Geometry check sheet. Reference: the model listing, model coordinates, mm. Face numbers are marked on the shaded views. A direction names the side the tool comes from. Give positions to 0.01 mm unless a question says otherwise; leave off trailing zeros. Loops run counter-clockwise (first coordinate to the right, second up) from the corner with the lowest first, then second, coordinate; pieces in that order, holes last. Notation, with made-up numbers: (-7, 33) -> (15, 33) arc R31 cw to (15, 61) -> close; hole circle Ø7 at (24.25, 66). An arc over 180 degrees is marked (long way). One line per item, written item: value. Start each with the question number.
(1) Scan lines: line 1 along X through (y, z) = (36.5, 28); line 2 along Y through (x, z) = (-22.5, 28); line 3 along Y through (x, z) = (21, 1.5). Record each from-to range of solid material in increasing order. Write a range as from..to.
(2) Tool access check on the marked faces 1, 2 and 3. Record the directions out of +Z, -Z, +X, -X, +Y, -Y that give a thin tool (end or side, any length) a straight path to the whole face; none if there is none.
(3) Draft check along Y on the marked faces 4, 5 and 6. Enter one of: pulls with the +Y half, pulls with the -Y half, needs draft (parallel to the pull), parting line crosses it, or undercut.
(4) Sectioned sample at B-B, the plane y = -69. Record the cut outline in (x, z).
(5) Gauge pin test, flat ends, axial feed: pin 1 Ø4 at (y, z) = (45, 14) entering from +X; pin 2 Ø4 at (x, y) = (-29, 64) entering from +Z; pin 3 Ø12 at (x, y) = (24.5, 66) entering from -Z; pin 4 Ø3 at (x, y) = (-10, 18.5) entering from -Z. Record the tip position at first contact, or that the pin passes through.
(6) Sectioned sample at C-C, the plane y = 1. Record the cut outline in (x, z), then the cut area to 3 significant figures.
(7) Sectioned sample at A-A, the plane x = 109. Record the cut outline in (y, z), then the cut area to 3 significant figures.
from build123d import *

# Parameters (mm, degrees)
F0_W      = 252.4125
F0_H      = 252.4125
F0_W_2    = 100.80625
F0_H_2    = 100.80625
F1_DEPTH  = 25.4
F2_W      = 100.80625
F2_H      = 100.80625
F3_DEPTH  = 6.35
F4_R      = 4
F4_R_2    = 1.7272
F5_DEPTH  = 6.35
F6_W      = 14.3500094
F6_H      = 31.75
F7_DEPTH  = 1.5875
F8_R      = 4
F9_DEPTH  = 6.35
F10_W     = 252.4125
F10_H     = 252.4125
F10_W_2   = 100.80625
F10_H_2   = 100.80625
F10_W_3   = 1.5875
F10_H_3   = 14.3500094
F11_DEPTH = 6.35


with BuildPart() as f1:
    # F0 (on Top) → F1 (new body)
    with BuildSketch(Plane.XY):
        Rectangle(F0_W, F0_H)
        Polygon((12.7, -12.7), (12.7, -119.85625), (-119.85625, -119.85625), (-119.85625, 12.7), (-12.7, 12.7), (-12.7, 119.85625), (119.85625, 119.85625), (119.85625, -12.7), align=None, mode=Mode.SUBTRACT)
        with Locations((69.453125, -69.453125)):
            Rectangle(F0_W_2, F0_H_2, mode=Mode.SUBTRACT)
        with Locations((-69.453125, 69.453125)):
            Rectangle(F0_W_2, F0_H_2, mode=Mode.SUBTRACT)
    extrude(amount=F1_DEPTH)

    # F2 (on face) → F3 (join)
    with BuildSketch(Plane.XY.offset(25.4)):
        Polygon((126.20625, -126.20625), (126.20625, 12.7), (119.85625, 12.7), (119.85625, -12.7), (12.7, -12.7), (12.7, -119.85625), (-12.7, -119.85625), (-12.7, -126.20625), align=None)
        with Locations((69.453125, -69.453125)):
            Rectangle(F2_W, F2_H, mode=Mode.SUBTRACT)
        Polygon((12.7, 126.20625), (-126.20625, 126.20625), (-126.20625, -12.7), (-119.85625, -12.7), (-119.85625, 12.7), (-12.7, 12.7), (-12.7, 119.85625), (12.7, 119.85625), align=None)
        with Locations((-69.453125, 69.453125)):
            Rectangle(F2_W, F2_H, mode=Mode.SUBTRACT)
        Polygon((12.7, 12.7), (12.7, 119.85625), (-12.7, 119.85625), (-12.7, 12.7), (-119.85625, 12.7), (-119.85625, -12.7), (-12.7, -12.7), (-12.7, -119.85625), (12.7, -119.85625), (12.7, -12.7), (119.85625, -12.7), (119.85625, 12.7), align=None)
        Polygon((-119.85625, -12.7), (-126.20625, -12.7), (-126.20625, -126.20625), (-12.7, -126.20625), (-12.7, -119.85625), (-119.85625, -119.85625), align=None)
        Polygon((126.20625, 126.20625), (12.7, 126.20625), (12.7, 119.85625), (119.85625, 119.85625), (119.85625, 12.7), (126.20625, 12.7), align=None)
    extrude(amount=F3_DEPTH)

    # F4 (on face) → F5 (cut, through all)
    with BuildSketch(Plane.YZ.offset(126.20625)):
        with Locations((107.91875, 12.7)):
            Circle(F4_R)
        with Locations((115.8875, 12.7)):
            Circle(F4_R_2)
        with Locations((99.95, 12.7)):
            Circle(F4_R_2)
        with Locations((44.41875, 12.7)):
            Circle(F4_R)
        with Locations((52.3875, 12.7)):
            Circle(F4_R_2)
        with Locations((36.45, 12.7)):
            Circle(F4_R_2)
    extrude(amount=-F5_DEPTH, mode=Mode.SUBTRACT)

    # F6 (on face) → F7 (join)
    with BuildSketch(Plane(origin=(-19.05, 0, 0), x_dir=(0, -1, 0), z_dir=(-1, 0, 0))):
        with Locations((-44.41875, 15.875)):
            Rectangle(F6_W, F6_H)
        with Locations((-107.91875, 15.875)):
            Rectangle(F6_W, F6_H)
    extrude(amount=F7_DEPTH)

    # F8 (on face) → F9 (cut, through all)
    with BuildSketch(Plane.YZ.offset(-12.7)):
        with Locations((44.41875, 12.7)):
            Circle(F8_R)
        with Locations((107.91875, 12.7)):
            Circle(F8_R)
    extrude(amount=-F9_DEPTH, mode=Mode.SUBTRACT)

    # F10 (on face) → F11 (join)
    with BuildSketch(Plane(origin=(0, 0, 0), x_dir=(1, 0, 0), z_dir=(0, 0, -1))):
        Rectangle(F10_W, F10_H)
        Polygon((-119.85625, -19.05), (-19.05, -19.05), (-19.05, -37.2437453), (-19.05, -51.5937547), (-19.05, -100.7437453), (-19.05, -115.0937547), (-19.05, -119.85625), (-119.85625, -119.85625), align=None, mode=Mode.SUBTRACT)
        Polygon((-119.85625, 119.85625), (12.7, 119.85625), (12.7, 12.7), (119.85625, 12.7), (119.85625, -119.85625), (-12.7, -119.85625), (-12.7, -12.7), (-119.85625, -12.7), align=None, mode=Mode.SUBTRACT)
        with Locations((69.453125, 69.453125)):
            Rectangle(F10_W_2, F10_H_2, mode=Mode.SUBTRACT)
        with Locations((69.453125, 69.453125)):
            Rectangle(F10_W_2, F10_H_2)
        Polygon((-19.05, -37.2437453), (-19.05, -19.05), (-119.85625, -19.05), (-119.85625, -119.85625), (-19.05, -119.85625), (-19.05, -115.0937547), (-20.6375, -115.0937547), (-20.6375, -100.7437453), (-19.05, -100.7437453), (-19.05, -51.5937547), (-20.6375, -51.5937547), (-20.6375, -37.2437453), align=None)
        with Locations((-19.84375, -44.41875)):
            Rectangle(F10_W_3, F10_H_3)
        with Locations((-19.84375, -107.91875)):
            Rectangle(F10_W_3, F10_H_3)
    extrude(amount=F11_DEPTH)


solid = f1.part
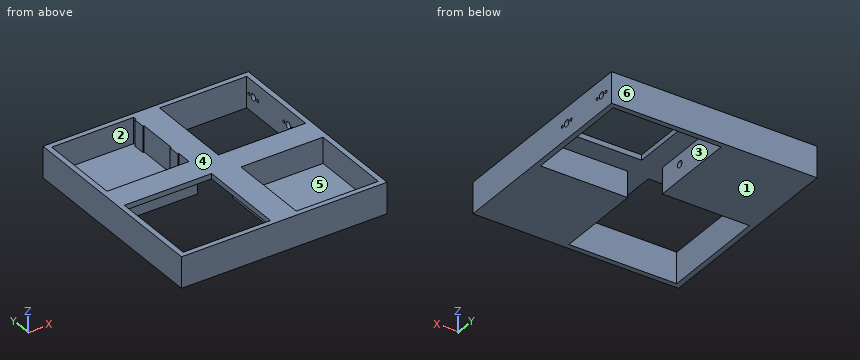
Calculated:
1. line 1: x = -126.21..-119.86, -19.05..12.7, 119.86..126.21
1. line 2: y = -126.21..-119.86, -12.7..19.05, 119.86..126.21
1. line 3: y = -126.21..-119.86, -19.05..-12.7, 119.86..126.21
2. face 1: -Z, +X, -X, +Y, -Y
2. face 2: +Z
2. face 3: -Z
3. face 4: needs draft
3. face 5: undercut
3. face 6: pulls with the +Y half
4. outline: (-126.21, -6.35) -> (-119.86, -6.35) -> (-119.86, 31.75) -> (-126.21, 31.75) -> close; (-12.7, 25.4) -> (12.7, 25.4) -> (12.7, -6.35) -> (126.21, -6.35) -> (126.21, 31.75) -> (119.86, 31.75) -> (119.86, 0) -> (19.05, 0) -> (19.05, 31.75) -> (-12.7, 31.75) -> close
5. pin 1: stops at x = -19.05
5. pin 2: stops at z = 0
5. pin 3: passes through
5. pin 4: stops at z = 25.4
6. outline: (-126.21, -6.35) -> (-119.86, -6.35) -> (-119.86, 25.4) -> (119.86, 25.4) -> (119.86, -6.35) -> (126.21, -6.35) -> (126.21, 31.75) -> (-126.21, 31.75) -> close
6. area: 2,010 mm2
7. outline: (-126.21, -6.35) -> (-12.7, -6.35) -> (-12.7, 25.4) -> (12.7, 25.4) -> (12.7, 31.75) -> (-19.05, 31.75) -> (-19.05, 0) -> (-119.86, 0) -> (-119.86, 31.75) -> (-126.21, 31.75) -> close; (119.86, -6.35) -> (126.21, -6.35) -> (126.21, 31.75) -> (119.86, 31.75) -> close
7. area: 1,530 mm2
